Can you work these out from the model? Positions are in its coordinate system, mm. A direction names the side the tool comes from. Round coordinates to 2 decimals unless told otherwise and drop trailing zeros. Loops run counter-clockwise (first coordinate to the right, second up) from the corner with the lowest first, then second, coordinate; pieces in that order, holes last.
Autodesk Inventor part; units mm, degrees
ref_plane "YZ Plane" through (0, 0, 0) normal (1, 0, 0) x (0, 1, 0)
ref_plane "XZ Plane" through (0, 0, 0) normal (0, 1, 0) x (-1, 0, 0)
ref_plane "XY Plane" through (0, 0, 0) normal (0, 0, 1) x (1, 0, 0)
sketch "Skizze1" plane through (0, 0, 0) normal (0, 0, 1) x (1, 0, 0)
  circle A0 centre (0, 0) radius 2.675
  circle A1 centre (0, 0) radius 5
  dimension "d0" = 5.35
  dimension "d3" = 10
extrude "Extrusion1" add sketch "Skizze1" along normal blind 20
sketch "Skizze2" plane through (0, 0, 0) normal (0, 0, -1) x (-1, 0, 0)
  circle A0 centre (0, 0) radius 2.675
  circle A1 centre (2.675, 0) radius 0.5
  circle A2 centre (0, 2.675) radius 0.5
  circle A3 centre (-2.675, 0) radius 0.5
  circle A4 centre (0, -2.675) radius 0.5
  point P0 (0.4978, -2.6283)
  point P1 (-0.4978, -2.6283)
  point P2 (2.6283, 0.4978)
  point P3 (2.6283, -0.4978)
  point P4 (-0.4978, 2.6283)
  point P5 (0.4978, 2.6283)
  dimension "d4" = 1
  dimension "d7" = 360
extrude "Extrusion2" add sketch "Skizze2" against normal blind 2 contours A0 A1 | A2 A0 | A0 A4 | A3 A0 | A0 A3 picked at (2.5116, 0.0962) picked at (0, 2.5049) picked at (0, -2.5049)
sketch "Skizze3" plane through (0, 0, 2) normal (0, 0, 1) x (1, 0, 0)
  circle A0 centre (0, 0) radius 2.675
  circle A1 centre (0, 0) radius 2.175
  arc A2 (-2.6283, -0.4978) -> (-2.6283, 0.4978) centre (-2.675, 0) ccw
extrude "Extrusion3" add sketch "Skizze3" along normal up to surface (18 mm away)
sketch "Skizze4" plane through (0, 0, 20) normal (0, 0, 1) x (1, 0, 0)
  circle A0 centre (0, 0) radius 5
  circle A1 centre (0, -5) radius 1
  circle A2 centre (5, 0) radius 1
  circle A3 centre (0, 5) radius 1
  circle A4 centre (-5, 0) radius 1
  point P0 (-0.995, 4.9)
  point P1 (0.995, 4.9)
  point P2 (4.9, 0.995)
  point P3 (4.9, -0.995)
  point P4 (0.995, -4.9)
  point P5 (-0.995, -4.9)
  point P6 (-4.9, -0.995)
  point P7 (-4.9, 0.995)
  dimension "d28" = 2
  dimension "d31" = 360
extrude "Extrusion4" cut sketch "Skizze4" against normal blind 10 contours A0 A2 | A3 A0 | A0 A1 | A4 A0 picked at (4.6729, -0.1921) picked at (0, 4.6592) picked at (0, -4.6592) picked at (-4.6592, 0)
chamfer "Fase6" distance 0.5 angle 45 4 edges at (0, 4, 10) (4, 0, 10) (0, -4, 10) (-4, 0, 10)
properties part number "Raspberry Pi Camera v.1 Focus Tool"
(1) For faces 4 (the flat face through (-1.6, -1.7, 2)), 5 (the flat face through (2, -2, 0)), 6 (the cylindrical face through (0, 4, 15)), 7 (the cylindrical face through (0, -4, 15)), 8 (the cylindrical face through (4, 0, 15)), which set-ups out of +Z, -Z, +X, -X, +Y, -Y let a thin tool reach every point of the face, with its end or its side?
Worked answers:
face 4: -Z
face 5: -Z, +X, -X, +Y, -Y
face 6: +Z, +Y
face 7: +Z, -Y
face 8: +Z, +X
(2) If we mould it in two halves opening along X, with no side actions, what happens to faces 1 (the cylindrical face through (-1.907, 1.876, 0.986)), 2 (the conical face through (4.36, 0.01, 10.14)), 3 (the cylindrical face through (-4, 0, 15))? For each: released by +X, released by -X, zero draft, split by the parting line, or undercut.
Worked answers:
face 1: undercut
face 2: released by +X
face 3: released by -X
(3) If we section it at D-D, the plane x = -3.75: List the corners of the cut face in (y, z) for me, then the cut area to 3 significant figures.
Worked answers:
outline: (-3.31, 0) - (3.31, 0) - (3.31, 20) - (-3.31, 20) - close
area: 132 mm2
(4) Will these pins go through, and if not, where does the flat tip stop? P1, Ø3, axis at x = 1, y = 2, coming from the -Z side; P2, Ø5, axis at x = -3.5, z = 5, coming from the +Y side; P3, Ø4, axis at y = 4, z = 14.5, coming from the -X side; P4, Ø2, axis at x = -1.5, z = 9.5, coming from the +Y side.
Worked answers:
P1: stops at z = 0
P2: stops at y = 4.9
P3: stops at x = -4.58
P4: stops at y = 4.97
(5) If we section it at A-A, the plane z = 12: List the corners of the cut face in (x, y) for me (3 decimals).
Worked answers:
outline: (-4.9, -0.995) arc R5 ccw to (-0.995, -4.9) arc R1 cw to (0.995, -4.9) arc R5 ccw to (4.9, -0.995) arc R1 cw to (4.9, 0.995) arc R5 ccw to (0.995, 4.9) arc R1 cw to (-0.995, 4.9) arc R5 ccw to (-4.9, 0.995) arc R1 cw to start; hole circle Ø4.35 at (0, 0)
(6) If I drill on line 1 (Y direction, x = 0, z = 12.25) (3 decimals); line 2 (Z direction, x = -1.25, y = -2.25); line 3 (Y direction, x = 0, z = 9) (3 decimals), over which ranges is the centre line in solid material (lowest first)?
Worked answers:
line 1: y = -4 to -2.175, 2.175 to 4
line 2: z = 2 to 20
line 3: y = -5 to -2.175, 2.175 to 5
(7) If we section it at B-B, the plane y = 1.75: List the corners of the cut face in (x, z) for me.
Worked answers:
outline: (-4.68, 0) - (-2.02, 0) - (-2.02, 2) - (-1.29, 2) - (-1.29, 20) - (-4.68, 20) - close; (1.29, 2) - (2.02, 2) - (2.02, 0) - (4.68, 0) - (4.68, 20) - (1.29, 20) - close
(8) If we section it at C-C, the plane z = 7: List the corners of the cut face in (x, y) for me (3 decimals), then the cut area to 3 significant figures.
Worked answers:
outline: circle Ø10 at (0, 0); hole circle Ø4.35 at (0, 0)
area: 63.7 mm2
